from build123d import *

# Parameters (mm, degrees)
SKETCH2_R           = 1.5
SKETCH2_R_2         = 4
SKETCH2_W           = 12.5
SKETCH2_H           = 20
BOSS_EXTRUDE1_DEPTH = 3.175
BOSS_EXTRUDE2_DEPTH = 3.175


with BuildPart() as part:
    # Sketch2 → Boss-Extrude1 (new body)
    with BuildSketch(Plane.XY):
        Polygon((-71.75862069, 50), (-71.75862069, 2), (74.24137931, 2), (74.24137931, 50), (69.808349218, 50), (69.808349218, 41), (55.808349218, 41), (55.808349218, 50), (52.24137931, 50), (52.24137931, 34), (44.24137931, 34), (44.24137931, 50), (39.953145567, 50), (39.953145567, 41), (28.953145567, 41), (28.953145567, 50), (5.35837424, 50), (5.35837424, 11.04586532), (-67.810407441, 11.04586532), (-67.810407441, 50), align=None)
        with Locations((23.74137931, 10)):
            Circle(SKETCH2_R, mode=Mode.SUBTRACT)
        with Locations((13.24137931, 10)):
            Circle(SKETCH2_R, mode=Mode.SUBTRACT)
        with Locations((57.871281099, 24)):
            Circle(SKETCH2_R_2, mode=Mode.SUBTRACT)
        with Locations((35.871281099, 24)):
            Circle(SKETCH2_R_2, mode=Mode.SUBTRACT)
        with Locations((18.49137931, 32)):
            Rectangle(SKETCH2_W, SKETCH2_H, mode=Mode.SUBTRACT)
    extrude(amount=BOSS_EXTRUDE1_DEPTH)

    # Sketch3 → Boss-Extrude2 (add)
    with BuildSketch(Plane(origin=(0, 0, 0), x_dir=(-1, 0, 0), z_dir=(0, 0, -1))):
        Polygon((-74.24137931, 50), (-76.24137931, 50), (-76.24137931, 0), (73.75862069, 0), (73.75862069, 50), (71.75862069, 50), (71.75862069, 2), (-74.24137931, 2), align=None)
    extrude(amount=-BOSS_EXTRUDE2_DEPTH)


solid = part.part
Check sheet for the modelled part. Datum: model origin and axes. Units: mm. A direction names the side the tool comes from. Round coordinates to 2 decimals unless told otherwise and drop trailing zeros. Loops run counter-clockwise (first coordinate to the right, second up) from the corner with the lowest first, then second, coordinate; pieces in that order, holes last. Notation, with made-up numbers: M 51,-40 L 94,-40 A33 cw 94,-6 Z; hole C 55,46 d2. An arc over 180 degrees is marked long. One line per item, written item: value.
(1) Access from +Z, -Z, +X, -X, +Y, -Y to the whole of each face (thin tool, end or side, straight path). Record for faces 1 (the face through (28.953, 45, 2)), 2 (the face through (76.241, 25, 2)).
Computed values:
face 1: +Z, -Z, +Y
face 2: +Z, -Z, +X, +Y, -Y
(2) Sectioned sample at A-A, the plane z = 2.6. Record the cut outline in (x, y), then the cut area to 3 significant figures.
Computed values:
outline: M -73.76,0 L 76.24,0 L 76.24,50 L 69.81,50 L 69.81,41 L 55.81,41 L 55.81,50 L 52.24,50 L 52.24,34 L 44.24,34 L 44.24,50 L 39.95,50 L 39.95,41 L 28.95,41 L 28.95,50 L 5.36,50 L 5.36,11.05 L -67.81,11.05 L -67.81,50 L -73.76,50 Z; hole C 13.24,10 d3; hole M 12.24,22 L 24.74,22 L 24.74,42 L 12.24,42 Z; hole C 23.74,10 d3; hole C 35.87,24 d8; hole C 57.87,24 d8
area: 3,930 mm^2
(3) Sectioned sample at C-C, the plane x = -36.5. Record the cut outline in (y, z) (3 decimals), then the cut area to 3 significant figures.
Computed values:
outline: M 0,0 L 11.046,0 L 11.046,3.175 L 0,3.175 Z
area: 35.1 mm^2
(4) Sectioned sample at B-B, the plane y = 24. Record the cut outline in (x, z) (3 decimals), then the cut area to 3 significant figures.
Computed values:
outline: M -73.759,0 L -67.81,0 L -67.81,3.175 L -73.759,3.175 Z; M 5.358,0 L 12.241,0 L 12.241,3.175 L 5.358,3.175 Z; M 24.741,0 L 31.871,0 L 31.871,3.175 L 24.741,3.175 Z; M 39.871,0 L 53.871,0 L 53.871,3.175 L 39.871,3.175 Z; M 61.871,0 L 76.241,0 L 76.241,3.175 L 61.871,3.175 Z
area: 153 mm^2
(5) Depth check by flat-ended pin: pin 1 Ø1 at (x, z) = (47, 2) entering from +Y. Enter the tip coordinate at first touch or a pass-through.
Computed values:
pin 1: stops at y = 34
(6) Release check for a two-part mould opening along Y. For faces 3 (the face through (61.687, 25.201, 1.565)), 4 (the face through (54, 50, 2)), 5 (the face through (19, 20, 0)) record: +Y half, -Y half, draft (parallel to the pull), parting line (faces both ways), or undercut.
Computed values:
face 3: undercut
face 4: +Y half
face 5: draft
(7) Thickness scan on line 1 (X direction, y = 40, z = 0.75); line 2 (Y direction, x = 24, z = 0.85); line 3 (X direction, y = 46, z = 0.7). Record the ranges inside material, lowest first.
Computed values:
line 1: x = -73.76 to -67.81, 5.36 to 12.24, 24.74 to 44.24, 52.24 to 76.24
line 2: y = 0 to 8.52, 11.48 to 22, 42 to 50
line 3: x = -73.76 to -67.81, 5.36 to 28.95, 39.95 to 44.24, 52.24 to 55.81, 69.81 to 76.24
